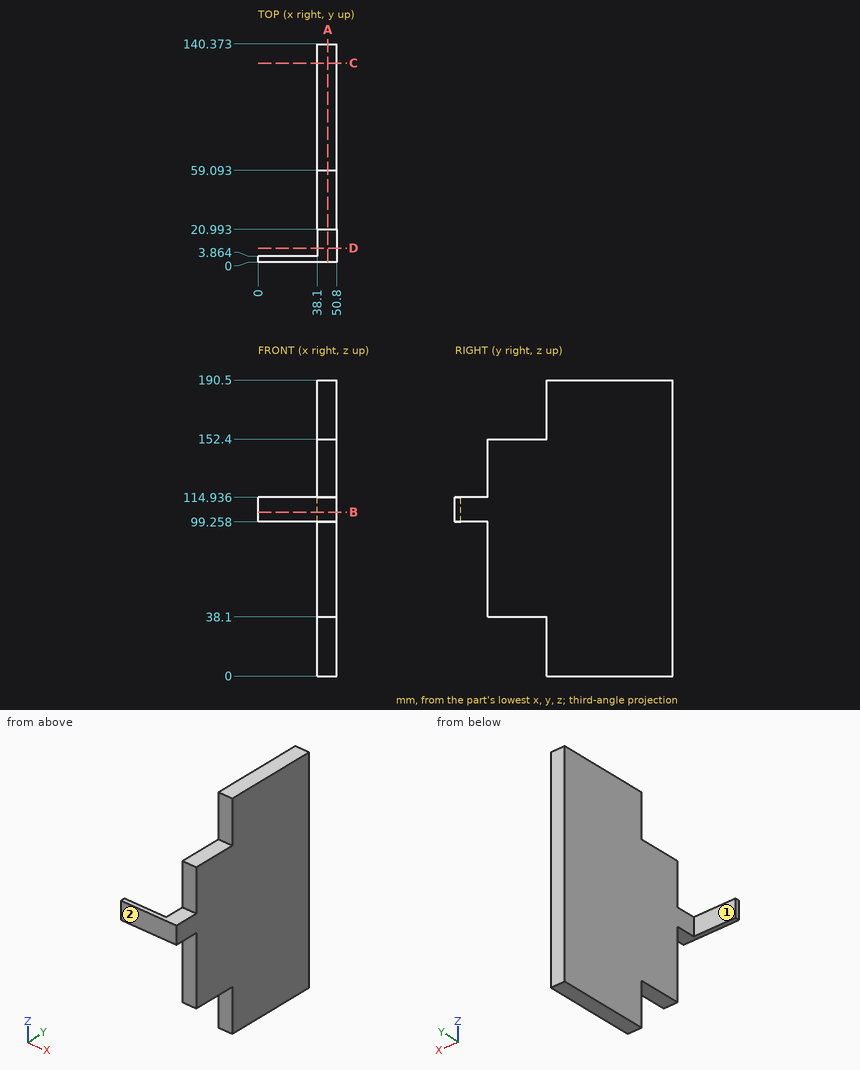
Answer from the drawing. Dimensions are ordinates in mm from the lowest x, y and z of the part. A direction names the side the tool comes from. Round coordinates to 2 decimals unless told otherwise and drop trailing zeros. Write each loop counter-clockwise with the first axis right and the second up, starting at its lowest first coordinate (ties: lowest second). Pieces come first, ordered by that corner, then holes. Notation, with made-up numbers: (-4, 62.25) -> (51, 62.25) arc R16 ccw to (51, 77.25) -> close; hole circle Ø11 at (-13.5, 47.25). An arc over 180 degrees is marked (long way). Write each question's results on one line, items separated by ' | '.
1) Which of the six approach directions +Z, -Z, +X, -X, +Y, -Y give full straight-line access (tool end or side, diameter ignored) to the marked faces 1 and 2?
Findings:
face 1: +Z, -Z, -X, +Y | face 2: +Z, -Z, +X, -X, -Y
2) The part is cut by section B-B (z = 105.5). Write down the section's boundary in (x, y) (1 decimal), and give its area (3 significant figures).
Findings:
outline: (0, 0) -> (50.8, 0) -> (50.8, 140.4) -> (38.1, 140.4) -> (38.1, 3.9) -> (0, 3.9) -> close | area: 1,930 mm²
3) The part is cut by section D-D (y = 9). Write down the section's boundary in (x, z), and give its area (3 significant figures).
Findings:
outline: (38.1, 99.26) -> (50.8, 99.26) -> (50.8, 114.94) -> (38.1, 114.94) -> close | area: 199 mm²
4) Flat-ended cylindrical pins translate along their axes: pin 1 (6.5 mm diameter, centred on x = 45, z = 13, fed in from -Y); pin 2 (14 mm diameter, centred on x = 45.5, y = 49, fed in from +Z); pin 3 (23 mm diameter, centred on x = 15.5, y = 14.5, fed in from -Z). Find the tip coordinate at first contact, or state that the pin passes through.
Findings:
pin 1: stops at y = 59.09 | pin 2: stops at z = 152.4 | pin 3: stops at z = 99.26
5) Consider line 1 along Y through (x, z) = (48, 146.5); line 2 along X through (y, z) = (26, 118); line 3 along Y through (x, z) = (38.5, 159.5). Determine where each line is inside the solid, lowest interval first. Write a range as [from, to].
Findings:
line 1: y = [20.99, 140.37] | line 2: x = [38.1, 50.8] | line 3: y = [59.09, 140.37]
6) The part is cut by section A-A (x = 45). Write down the section's boundary in (y, z).
Findings:
outline: (0, 99.26) -> (20.99, 99.26) -> (20.99, 38.1) -> (59.09, 38.1) -> (59.09, 0) -> (140.37, 0) -> (140.37, 190.5) -> (59.09, 190.5) -> (59.09, 152.4) -> (20.99, 152.4) -> (20.99, 114.94) -> (0, 114.94) -> close
7) The part is cut by section C-C (y = 128). Write down the section's boundary in (x, z).
Findings:
outline: (38.1, 0) -> (50.8, 0) -> (50.8, 190.5) -> (38.1, 190.5) -> close
